Here's how the part is built. I have some questions about the finished solid (model axes, mm). Face numbers are marked on the shaded views. A direction names the side the tool comes from. Coordinates: 2 decimals unless noted, no trailing zeros. Write each loop counter-clockwise with the first axis right and the second up, starting at its lowest first coordinate (ties: lowest second). Pieces come first, ordered by that corner, then holes. Notation, with made-up numbers: (24.5, 17) -> (44.5, 17) arc R22 ccw to (44.5, 43) -> close; hole circle Ø3 at (76.25, -18.5). An arc over 180 degrees is marked (long way). Answer in a Markdown table with one row per item. Add a question column.
from build123d import *
from build123d.topology import SkipClean

# Parameters (mm, degrees)
SKETCH5_R           = 139.7
BOSS_EXTRUDE3_DEPTH = 12.7
SKETCH6_R           = 38.1
SKETCH6_R_2         = 19.05
BOSS_EXTRUDE4_DEPTH = 63.5
CUT_EXTRUDE3_START  = -63.5
SKETCH7_R           = 19.05
CUT_EXTRUDE3_DEPTH  = 63.5
BOSS_EXTRUDE5_DEPTH = 165.1
SKETCH10_R          = 139.7
BOSS_EXTRUDE6_DEPTH = 6.35
SKETCH11_R          = 101.6
CUT_EXTRUDE4_DEPTH  = 6.35


with BuildPart() as part:
    # Sketch5 → Boss-Extrude3 (new body)
    with BuildSketch(Plane(origin=(0, 0, 0), x_dir=(0, 0, -1), z_dir=(1, 0, 0))):
        Circle(SKETCH5_R)
    extrude(amount=BOSS_EXTRUDE3_DEPTH)

    # Sketch6 → Boss-Extrude4 (add)
    with BuildSketch(Plane.ZY):
        Circle(SKETCH6_R)
        Circle(SKETCH6_R_2, mode=Mode.SUBTRACT)
    extrude(amount=BOSS_EXTRUDE4_DEPTH)

    # Sketch7 → Cut-Extrude3 (cut)
    with BuildSketch(Plane.ZY.offset(CUT_EXTRUDE3_START)):
        with Locations(Location((0, 0, 0), (0, 0, 180))):
            Circle(SKETCH7_R)
    extrude(amount=CUT_EXTRUDE3_DEPTH, mode=Mode.SUBTRACT)

    # Sketch9 → Boss-Extrude5 (add)
    with SkipClean():  # the faces are left unmerged after this step: merging them gives an invalid solid
        with BuildSketch(Plane(origin=(12.7, 0, 0), x_dir=(0, 0, -1), z_dir=(1, 0, 0))):
            with BuildLine():
                Line((-139.7, 0), (-76.2, 0))
                Line((-76.2, 0), (-76.2, 6.35))
                Line((-76.2, 6.35), (-135.741554433, 6.35))
                ThreePointArc((-135.741554433, 6.35), (-131.694050685, 33.507747077), (-122.269799969, 59.297454545))
                Line((-122.269799969, 59.297454545), (-125.697925202, 60.96))
                ThreePointArc((-125.697925202, 60.96), (-136.154489736, 31.2737098), (-139.7, 0))
            make_face()
            with BuildLine():
                Line((-115.641871216, -78.377596428), (-112.488002001, -76.240025616))
                ThreePointArc((-112.488002001, -76.240025616), (-94.865585535, -97.296519882), (-73.370038531, -114.380634489))
                Line((-73.370038531, -114.380634489), (-43.599261314, -62.816135768))
                Line((-43.599261314, -62.816135768), (-38.1, -65.991135768))
                Line((-38.1, -65.991135768), (-69.85, -120.983748909))
                ThreePointArc((-69.85, -120.983748909), (-95.161072026, -102.276392051), (-115.641871216, -78.377596428))
            make_face()
            with BuildLine():
                Line((10.056053986, -139.337596428), (9.781797968, -135.537480161))
                ThreePointArc((9.781797968, -135.537480161), (36.82846515, -130.804266959), (62.371515903, -120.730634489))
                Line((62.371515903, -120.730634489), (32.600738686, -69.166135768))
                Line((32.600738686, -69.166135768), (38.1, -65.991135768))
                Line((38.1, -65.991135768), (69.85, -120.983748909))
                ThreePointArc((69.85, -120.983748909), (40.993417711, -133.550101851), (10.056053986, -139.337596428))
            make_face()
            with BuildLine():
                Line((125.697925202, -60.96), (122.269799969, -59.297454545))
                ThreePointArc((122.269799969, -59.297454545), (131.694050685, -33.507747077), (135.741554433, -6.35))
                Line((135.741554433, -6.35), (76.2, -6.35))
                Line((76.2, -6.35), (76.2, 0))
                Line((76.2, 0), (139.7, 0))
                ThreePointArc((139.7, 0), (136.154489736, -31.2737098), (125.697925202, -60.96))
            make_face()
            with BuildLine():
                Line((115.641871216, 78.377596428), (112.488002001, 76.240025616))
                ThreePointArc((112.488002001, 76.240025616), (94.865585535, 97.296519882), (73.370038531, 114.380634489))
                Line((73.370038531, 114.380634489), (43.599261314, 62.816135768))
                Line((43.599261314, 62.816135768), (38.1, 65.991135768))
                Line((38.1, 65.991135768), (69.85, 120.983748909))
                ThreePointArc((69.85, 120.983748909), (95.161072026, 102.276392051), (115.641871216, 78.377596428))
            make_face()
            with BuildLine():
                Line((-10.056053986, 139.337596428), (-9.781797968, 135.537480161))
                ThreePointArc((-9.781797968, 135.537480161), (-36.82846515, 130.804266959), (-62.371515903, 120.730634489))
                Line((-62.371515903, 120.730634489), (-32.600738686, 69.166135768))
                Line((-32.600738686, 69.166135768), (-38.1, 65.991135768))
                Line((-38.1, 65.991135768), (-69.85, 120.983748909))
                ThreePointArc((-69.85, 120.983748909), (-40.993417711, 133.550101851), (-10.056053986, 139.337596428))
            make_face()
        extrude(amount=BOSS_EXTRUDE5_DEPTH)

    # Sketch10 → Boss-Extrude6 (add)
    with SkipClean():  # the faces are left unmerged after this step: merging them gives an invalid solid
        with BuildSketch(Plane(origin=(177.8, 0, 0), x_dir=(0, 0, -1), z_dir=(1, 0, 0))):
            Circle(SKETCH10_R)
        extrude(amount=BOSS_EXTRUDE6_DEPTH)

    # Sketch11 → Cut-Extrude4 (cut)
    with SkipClean():  # the faces are left unmerged after this step: merging them gives an invalid solid
        with BuildSketch(Plane(origin=(184.15, 0, 0), x_dir=(0, 0, -1), z_dir=(1, 0, 0))):
            Circle(SKETCH11_R)
        extrude(amount=-CUT_EXTRUDE4_DEPTH, mode=Mode.SUBTRACT)


solid = part.part
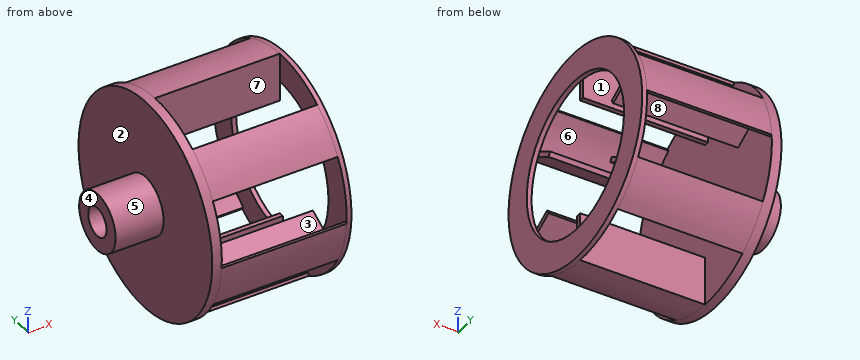
Q1. Imagine slicing it at A-A on z = 0. Please give me the cut outline in (x, y).
Q2. I need wall thicknesses on line 1 (Y direction, x = 3, z = 0); line 2 (X direction, y = -75, z = -108); line 3 (Z direction, x = 119.5, y = 92.5). Which ranges of each line are inside material? Lowest first, please. Write a range as [from, to].
Q3. For the marked faces 1, 2, 3 and 4, which set-ups out of +Z, -Z, +X, -X, +Y, -Y let a thin tool reach every point of the face, with its end or its side?
Q4. I'm going to push flat-ended pins straight in: P1, Ø1, axis at x = 102, z = -97, coming from the -Y side; P2, Ø14.5, axis at y = -75, z = -40, coming from the +X side; P3, Ø6, axis at x = 59.5, y = -17, coming from the -Z side; P4, Ø7, axis at x = 108, y = -3, coming from the +Z side. Where does each tip first touch, or does it pass through?
Q5. Imagine slicing it at C-C on x = 71.5. State how many separate pieces and enclosed holes the cut face has, plus the area to 3 significant figures.
Q6. If we mould it in two halves opening along Z, with no side actions, what happens to the marked faces 5, 6, 7 and 8? For each: pulls with the +Z half, pulls with the -Z half, needs draft (parallel to the pull), parting line crosses it, or undercut.
Q7. Imagine slicing it at B-B on y = -12. Please give me the cut outline in (x, z), plus the area to 3 significant figures.
Result sheet:
| question | item | result |
|---|---|---|
| 1 | outline | (-63.5, -38.1) -> (0, -38.1) -> (0, -139.7) -> (12.7, -139.7) -> (12.7, -19.05) -> (-63.5, -19.05) -> close; (-63.5, 19.05) -> (12.7, 19.05) -> (12.7, 139.7) -> (0, 139.7) -> (0, 38.1) -> (-63.5, 38.1) -> close; (177.8, -139.7) -> (184.15, -139.7) -> (184.15, -101.6) -> (177.8, -101.6) -> close; (177.8, 101.6) -> (184.15, 101.6) -> (184.15, 139.7) -> (177.8, 139.7) -> close |
| 2 | line 1 | y = [-139.7, -19.05], [19.05, 139.7] |
| 2 | line 2 | x = [0, 12.7], [177.8, 184.15] |
| 2 | line 3 | z = [-104.69, -99.55], [-60.74, -53.4], [46.07, 53.4] |
| 3 | face 1 | -Z |
| 3 | face 2 | -X |
| 3 | face 3 | none |
| 3 | face 4 | +Z, -Z, -X, +Y, -Y |
| 4 | P1 | stops at y = -6.35 |
| 4 | P2 | stops at x = 177.8 |
| 4 | P3 | stops at z = -139 |
| 4 | P4 | stops at z = 139.7 |
| 5 | separate pieces | 6 |
| 5 | enclosed holes | 0 |
| 5 | area | 3,690 mm^2 |
| 6 | face 5 | parting line crosses it |
| 6 | face 6 | undercut |
| 6 | face 7 | needs draft |
| 6 | face 8 | undercut |
| 7 | outline | (-63.5, -36.16) -> (0, -36.16) -> (0, -139.18) -> (184.15, -139.18) -> (184.15, -100.89) -> (177.8, -100.89) -> (177.8, -135.36) -> (12.7, -135.36) -> (12.7, -14.8) -> (-63.5, -14.8) -> close; (-63.5, 14.8) -> (12.7, 14.8) -> (12.7, 139.18) -> (0, 139.18) -> (0, 36.16) -> (-63.5, 36.16) -> close; (177.8, 100.89) -> (184.15, 100.89) -> (184.15, 139.18) -> (177.8, 139.18) -> close |
| 7 | area | 6,990 mm^2 |
